```python
from build123d import *

# Parameters (mm, degrees)
F1_DEPTH = 20
F2_T     = -6
F4_DEPTH = 40.001
F5_R     = 8
F5_W     = 39.5979797464
F5_H     = 28
F6_DEPTH = 6
F7_W     = 28
F7_H     = 28
F8_DEPTH = 143.1345136524


with BuildPart() as f1:
    # F0 (on Top) → F1 (new body, symmetric)
    with BuildSketch(Plane.XY):
        with BuildLine():
            Line((-20, 32), (-20, 0))
            Line((-20, 0), (20, 0))
            ThreePointArc((20, 0), (23.5147186258, 8.4852813742), (32, 12))
            Line((32, 12), (120, 12))
            Line((120, 12), (80, 52))
            Line((80, 52), (0, 52))
            ThreePointArc((0, 52), (-14.1421356237, 46.1421356237), (-20, 32))
        make_face()
        Polygon((80, 52), (120, 12), (120, 52), align=None)
    extrude(amount=F1_DEPTH, both=True)

    # F2
    f2_openings = [f1.faces().sort_by_distance(p)[0] for p in [
        (0, 0, 0),
        (120, 32, 0),
    ]]
    offset(amount=F2_T, openings=f2_openings)

    # F3 (on face) → F4 (cut, through all)
    with BuildSketch(Plane.XZ.offset(-12)):
        Polygon((80, 20), (120, -20), (120, 20), align=None)
    extrude(amount=-F4_DEPTH, mode=Mode.SUBTRACT)

    # F5 (on face) → F6 (join)
    with BuildSketch(Plane(origin=(50, 0, 50), x_dir=(0.7071067812, 0, -0.7071067812), z_dir=(0.7071067812, 0, 0.7071067812))):
        with BuildLine():
            Line((106.4730738116, 64), (25.7106781187, 64))
            ThreePointArc((25.7106781187, 64), (11.8542716581, 56), (11.8542716581, 40))
            Line((11.8542716581, 40), (32.0615310797, 5))
            ThreePointArc((32.0615310797, 5), (35.7217851176, 1.3397459622), (40.7217851176, 0))
            Line((40.7217851176, 0), (115.7106781187, 0))
            ThreePointArc((115.7106781187, 0), (129.5670845792, 8), (129.5670845792, 24))
            Line((129.5670845792, 24), (106.4730738116, 64))
        make_face()
        with Locations((115.7106781187, 16)):
            Circle(F5_R, mode=Mode.SUBTRACT)
        with Locations((25.7106781187, 48)):
            Circle(F5_R, mode=Mode.SUBTRACT)
        with Locations((70.7106781187, 32)):
            Rectangle(F5_W, F5_H, mode=Mode.SUBTRACT)
    extrude(amount=-F6_DEPTH)

    # F7 (on Right) → F8 (cut, through all)
    with BuildSketch(Plane.YZ):
        with Locations((32, 0)):
            Rectangle(F7_W, F7_H)
    extrude(amount=F8_DEPTH, mode=Mode.SUBTRACT)


solid = f1.part
```
Read the model definition and answer for the solid it produces. Units are mm, in the model's axes. A direction names the side the tool comes from. Give positions to 0.01 mm unless a question says otherwise; leave off trailing zeros. Loops run counter-clockwise (first coordinate to the right, second up) from the corner with the lowest first, then second, coordinate; pieces in that order, holes last.
Item 1: The mould has two halves that part along X. Classify faces 5 (the flat face through (-20, 16, 0)), 6 (the flat face through (95.153, 11.115, -3.639)), 7 (the flat face through (25, 26, 20)): released by +X, released by -X, zero draft, split by the parting line, or undercut.
Item 2: Find the intervals of material crossed by line 1 along Y through (x, z) = (40, 10.5); line 2 along Z through (x, y) = (-2, 42.5); line 3 along Y through (x, z) = (88.5, 7.5), in increasing order.
Item 3: The part is cut by section D-D (y = 42.5). Write down the section's boundary in (x, z), and give its area (3 significant figures).
Item 4: The part is cut by section B-B (x = 35). Write down the section's boundary in (y, z).
Item 5: For faces 1 (the flat face through (45, 46, 0)), 2 (the cylindrical face through (19.133, 12.587, 0.196)), 3 (the cylindrical face through (73.123, 1.377, 22.694)), 4 (the cylindrical face through (23.42, 8.39, 0.28)), determine the directions among +Z, -Z, +X, -X, +Y, -Y from which every point of the face is accessible in a straight line to the end or side of a thin tool.
Item 6: Each of these flat-tipped pins is pushed along its axis until it touches: pin 1 Ø2 at (x, y) = (119, 24) entering from +Z; pin 2 Ø4 at (x, y) = (71, 15.5) entering from +Z; pin 3 Ø6 at (y, z) = (47, -28) entering from +X. Where does it stop, or does it pass through?
Item 7: The part is cut by section A-A (y = 10). Write down the section's boundary in (x, z), and give its area (3 significant figures).
Item 8: The part is cut by section C-C (z = -7). Write down the section's boundary in (x, y), and give its area (3 significant figures).
Taken from the geometry:
1. face 5: released by -X
1. face 6: undercut
1. face 7: zero draft
2. line 1: y = 12 to 18, 46 to 52
2. line 2: z = -20 to -14, 14 to 20
2. line 3: y = 0 to 18, 46 to 64
3. outline: (-17.02, -20) - (111.51, -20) - (129.82, -38.31) - (134.07, -34.07) - (114, -14) - (-9.26, -14) - (-9.26, 14) - (86, 14) - (72.29, 27.71) - (68.05, 23.47) - (71.51, 20) - (-17.02, 20) - close; (53.31, 38.2) - (59.83, 31.69) - (64.07, 35.93) - (57.56, 42.44) - close
3. area: 1,860 mm2
4. outline: (12, -20) - (52, -20) - (52, 20) - (12, 20) - close; hole (18, -14) - (46, -14) - (46, 14) - (18, 14) - close
5. face 1: +X
5. face 2: none
5. face 3: +Z, -Y
5. face 4: +Z, -Z, -Y
6. pin 1: stops at z = -18
6. pin 2: stops at z = 31
6. pin 3: stops at x = 131
7. outline: (-20, -20) - (25.37, -20) - (25.37, 20) - (-20, 20) - close; (66.39, 25.13) - (123.84, -32.32) - (128.08, -28.08) - (70.63, 29.37) - close; (131.32, -39.8) - (138.07, -46.55) - (142.31, -42.31) - (135.56, -35.56) - close; hole (-14, -14) - (17.03, -14) - (17.03, 14) - (-14, 14) - close
7. area: 1,490 mm2
8. outline: (-20, 0) - (-14, 0) - (-14, 32) arc R14 cw to (0, 46) - (107, 46) - (107, 64) - (98.51, 64) - (98.51, 52) - (0, 52) arc R20 ccw to (-20, 32) - close; (14, 0) - (20, 0) arc R12 cw to (32, 12) - (98.51, 12) - (98.51, 0) - (107, 0) - (107, 18) - (32, 18) arc R18 ccw to start
8. area: 1,790 mm2
